Check sheet for the modelled part. Datum: model origin and axes. Units: mm. A direction names the side the tool comes from. Give positions to 0.01 mm unless a question says otherwise; leave off trailing zeros. Loops run counter-clockwise (first coordinate to the right, second up) from the corner with the lowest first, then second, coordinate; pieces in that order, holes last. Notation, with made-up numbers: (13, 61) - (41, 61) arc R38 ccw to (41, 99) - close; hole circle Ø6 at (-36.75, 51). An arc over 180 degrees is marked (long way). Use CSV: the item, a comma, the result in double quotes.
from build123d import *

# Parameters (mm, degrees)
F1_DEPTH       = 3
F2_D           = 3.4
F2_CSINK_D     = 6.3
F2_CSINK_ANGLE = 90
F3_R           = 8
F4_DEPTH       = 13
F5_R           = 5
F6_DEPTH       = 14
F7_R           = 4.5
F8_DEPTH       = 16
F9_SIZE        = 1.5
F10_SIZE       = 0.49999


# Not quite as in the source:
# - a fillet or chamfer is up to 0.001 mm smaller than in the source, because OpenCascade refuses the exact size


with BuildPart() as f1:
    # F0 (on Top) → F1 (new body)
    with BuildSketch(Plane.XY):
        with BuildLine():
            Line((9.7979589711, 10), (-9.7979589711, 10))
            ThreePointArc((-9.7979589711, 10), (-14, 0), (-9.7979589711, -10))
            Line((-9.7979589711, -10), (9.7979589711, -10))
            ThreePointArc((9.7979589711, -10), (14, 0), (9.7979589711, 10))
        make_face()
    extrude(amount=F1_DEPTH)

    # F2 (through all)
    with Locations(Plane(origin=(0, 0, 0), x_dir=(1, 0, 0), z_dir=(0, 0, -1))):
        with Locations((-10, 0), (10, 0)):
            CounterSinkHole(F2_D / 2, F2_CSINK_D / 2, counter_sink_angle=F2_CSINK_ANGLE)

    # F3 (on face) → F4 (join)
    with BuildSketch(Plane.XY.offset(3)):
        Circle(F3_R)
    extrude(amount=F4_DEPTH)

    # F5 (on face) → F6 (join)
    with BuildSketch(Plane.XY.offset(16)):
        Circle(F5_R)
    extrude(amount=F6_DEPTH)

    # F7 (on face) → F8 (join)
    with BuildSketch(Plane.XY.offset(30)):
        Circle(F7_R)
    extrude(amount=F8_DEPTH)

    # F9
    f9_edges = [f1.edges().sort_by_distance(p)[0] for p in [
        (-4.5, 0, 46),
    ]]
    chamfer(f9_edges, length=F9_SIZE)

    # F10 (size 0.5 in the source; OpenCascade refuses exactly that, so slightly less here)
    f10_edges = [f1.edges().sort_by_distance(p)[0] for p in [
        (-5, 0, 30),
        (0, -10, 3),
        (14, 0, 3),
        (0, 10, 3),
        (-14, 0, 3),
        (-14, 0, 0),
        (0, -10, 0),
        (14, 0, 0),
        (0, 10, 0),
        (-8, 0, 16),
    ]]
    chamfer(f10_edges, length=F10_SIZE)


solid = f1.part
1. Scan lines: line 1 along Y through (x, z) = (-10, 2.2); line 2 along Y through (x, z) = (10, 2.65); line 3 along Z through (x, y) = (-3.25, -7.75). Record each from-to range of solid material in increasing order.
Completed:
line 1,"y = -9.8 to -1.7, 1.7 to 9.8"
line 2,"y = -9.58 to -1.7, 1.7 to 9.58"
line 3,"z = 0 to 3"
2. Set-up check for faces 1 (the face through (-13.635, 0.152, 0.135)), 2 (the face through (5, -2, 16)): record each of +Z, -Z, +X, -X, +Y, -Y from which the full face is reachable in a straight line by a thin tool's end or side.
Completed:
face 1,"-Z, -X"
face 2,"+Z"
3. Sectioned sample at C-C, the plane z = 36. Record the boundary of the cut face in (x, y), and give its area (3 significant figures).
Completed:
outline,"circle Ø9 at (0, 0)"
area,"63.6 mm²"
4. Release check for a two-part mould opening along Y. For faces 3 (the face through (6, -6, 3)), 4 (the face through (8.43, 0.65, 2.24)), 5 (the face through (13.635, -0.152, 0.135)) record: released by +Y, released by -Y, zero draft, split by the parting line, or undercut.
Completed:
face 3,"zero draft"
face 4,"undercut"
face 5,"split by the parting line"
5. Go/stop test with flat-tipped pins: pin 1 Ø2 at (y, z) = (-3, 34) entering from -X; pin 2 Ø5.5 at (x, y) = (10, 0) entering from +Z; pin 3 Ø3 at (x, z) = (-5.5, 23.5) entering from +Y. Record where each tip stops, or that it passes through.
Completed:
pin 1,"stops at x = -4.03"
pin 2,"stops at z = 16"
pin 3,"stops at y = 3"
6. Sectioned sample at A-A, the plane y = 0. State how many separate pieces and enclosed holes the cut face has, and give its area (3 significant figures).
Completed:
separate pieces,"3"
enclosed holes,"0"
area,"548 mm²"
